Input: part model. Units: mm. Frame: model coordinates. Give positions to 0.01 mm unless a question says otherwise; leave off trailing zeros. Order: outer loops, then holes, each group sorted by start corner. A loop starts at its lowest first (then second) coordinate and runs counter-clockwise, first axis right, second up.
```python
from build123d import *

# Parameters (mm, degrees)
F0_W     = 50.8
F0_H     = 50.8
F1_DEPTH = 12.7
F2_R     = 2.54
F2_R_2   = 12.7
F3_DEPTH = 25.146


with BuildPart() as f1:
    # F0 (on Top) → F1 (new body)
    with BuildSketch(Plane.XY):
        Rectangle(F0_W, F0_H)
    extrude(amount=F1_DEPTH)

    # F2 (on face) → F3 (cut)
    with BuildSketch(Plane.XY.offset(12.7)):
        with Locations((17.78, 17.78)):
            Circle(F2_R)
        with Locations((17.78, -17.78)):
            Circle(F2_R)
        with Locations((-17.78, 17.78)):
            Circle(F2_R)
        with Locations((-17.78, -17.78)):
            Circle(F2_R)
        Circle(F2_R_2)
    extrude(amount=-F3_DEPTH, mode=Mode.SUBTRACT)


solid = f1.part
```
1) Pull-direction query (X, two-part tool) for faces 1 (the face through (-25.4, 0, 6)), 2 (the face through (-18.11, -15.26, 6.44)), 3 (the face through (-6, 12, 0)), 4 (the face through (-2.75, -12.4, 6.44)); classes: pulls with the +X half, pulls with the -X half, needs draft (parallel to the pull), parting line crosses it, or undercut.
2) Line query: probe 1 along Y at (x, z) = (-17.78, 10); probe 2 along X at (y, z) = (-19.5, 1.25); probe 3 along Y at (x, z) = (-17, 3.5). Output: solid intervals per line, ascending.
3) Cut plane A-A (y = -17.78). Return the cut outline in (x, z).
4) Cut plane C-C (x = -7.5). Return the cut outline in (y, z), then the cut area to 3 significant figures.
5) Cut plane B-B (z = 8). Return the cut outline in (x, y).
6) First-contact query: P1, Ø3, axis at x = 17.78, y = -17.78, coming from the +Z side. Flat tip, straight axial feed; report the tip coordinate or a pass-through.
7) Cut plane D-D (y = 0). Return the cut outline in (x, z).
Geometry says:
1. face 1: pulls with the -X half
1. face 2: undercut
1. face 3: needs draft
1. face 4: undercut
2. probe 1: y = -25.4 to -20.32, -15.24 to 15.24, 20.32 to 25.4
2. probe 2: x = -25.4 to -19.65, -15.91 to 15.91, 19.65 to 25.4
2. probe 3: y = -25.4 to -20.2, -15.36 to 15.36, 20.2 to 25.4
3. outline: (-25.4, 0) - (-20.32, 0) - (-20.32, 12.7) - (-25.4, 12.7) - close; (-15.24, 0) - (15.24, 0) - (15.24, 12.7) - (-15.24, 12.7) - close; (20.32, 0) - (25.4, 0) - (25.4, 12.7) - (20.32, 12.7) - close
4. outline: (-25.4, 0) - (-10.25, 0) - (-10.25, 12.7) - (-25.4, 12.7) - close; (10.25, 0) - (25.4, 0) - (25.4, 12.7) - (10.25, 12.7) - close
4. area: 385 mm2
5. outline: (-25.4, -25.4) - (25.4, -25.4) - (25.4, 25.4) - (-25.4, 25.4) - close; hole circle Ø5.08 at (-17.78, -17.78); hole circle Ø5.08 at (-17.78, 17.78); hole circle Ø25.4 at (0, 0); hole circle Ø5.08 at (17.78, -17.78); hole circle Ø5.08 at (17.78, 17.78)
6. P1: passes through
7. outline: (-25.4, 0) - (-12.7, 0) - (-12.7, 12.7) - (-25.4, 12.7) - close; (12.7, 0) - (25.4, 0) - (25.4, 12.7) - (12.7, 12.7) - close
